The model under review builds one solid part; all positions refer to its coordinate system, in mm. A direction names the side the tool comes from. Round coordinates to 2 decimals unless told otherwise and drop trailing zeros. Loops run counter-clockwise (first coordinate to the right, second up) from the corner with the lowest first, then second, coordinate; pieces in that order, holes last. Notation, with made-up numbers: (54.25, -19.5) -> (63.25, -19.5) arc R19 ccw to (63.25, 9.5) -> close; hole circle Ø11 at (32.5, 19.25). An arc over 180 degrees is marked (long way). Write each question's results on one line, items separated by ' | '. Start each with the question number.
Item 1: Clearance check with a flat-ended pin moving along its axis: pin 1 Ø1.9 at (x, z) = (-10, 22) entering from -Y. State where the tip first meets the part, or that it passes through.
Item 2: Mouldability with a two-part tool opening along X and no side actions: class faces 1 (the flat face through (30, 1, 0)), 2 (the flat face through (0, 1, -12.05)), 3 (the cylindrical face through (-26.58, 1.42, -21.39)) as pulls with the +X half, pulls with the -X half, needs draft (parallel to the pull), parting line crosses it, or undercut.
Item 3: We need section B-B (x = 10). Give the boundary of the cut face in (y, z), and give its area (3 significant figures).
Item 4: We need section D-D (x = -1). Give the boundary of the cut face in (y, z), and give its area (3 significant figures).
Item 5: Tool access review of faces 4 (the cylindrical face through (15.009, 1.38, 11.537)), 5 (the flat face through (0, 1, 25)): name each direction out of +Z, -Z, +X, -X, +Y, -Y from which nothing blocks a thin tool from reaching the whole face with its end or side.
Item 6: For L1, parallel to Z at x = 10, y = 1; L2, parallel to Z at x = -7, y = 0.35; L3, parallel to X at y = 0.1, z = 21, list the stretches that pass through material, from the lowest coordinate up. Write a range as from..to.
Item 7: We need section A-A (z = 8). Give the boundary of the cut face in (x, y), and give its area (3 significant figures).
Item 8: We need section C-C (y = 0.45). Give the number of separate pieces and of enclosed holes in the cut face, and give its area (3 significant figures).
from build123d import *

# Parameters (mm, degrees)
SKETCH_1_W          = 60
SKETCH_1_H          = 50
SKETCH_1_W_2        = 29.5
SKETCH_1_H_2        = 22.5
EXTRUDE_1_DEPTH     = 2.8
SKETCH_8_R          = 1.55
CUT_EXTRUDE_2_DEPTH = 10
FILLET_1_R          = 1
FILLET_2_R          = 12
CUT_EXTRUDE_3_DEPTH = 10


with BuildPart() as part:
    # 草图1 → 凸台-拉伸1 (new body)
    with BuildSketch(Plane(origin=(0, 0, 0), x_dir=(1, 0, 0), z_dir=(0, 1, 0))):
        Rectangle(SKETCH_1_W, SKETCH_1_H)
        Rectangle(SKETCH_1_W_2, SKETCH_1_H_2, mode=Mode.SUBTRACT)
    extrude(amount=EXTRUDE_1_DEPTH)

    # 草图8 → 切除-拉伸2 (cut)
    with BuildSketch(Plane.XZ):
        with Locations((27, 8)):
            Circle(SKETCH_8_R)
        with Locations((10, 22)):
            Circle(SKETCH_8_R)
        with Locations((-10, 22)):
            Circle(SKETCH_8_R)
        with Locations((-27, 8)):
            Circle(SKETCH_8_R)
        with Locations((-27, -8)):
            Circle(SKETCH_8_R)
        with Locations((-10, -22)):
            Circle(SKETCH_8_R)
        with Locations((10, -22)):
            Circle(SKETCH_8_R)
        with Locations((27, -8)):
            Circle(SKETCH_8_R)
    extrude(amount=-CUT_EXTRUDE_2_DEPTH, mode=Mode.SUBTRACT)

    # 圆角1
    fillet_1_edges = [part.edges().sort_by_distance(p)[0] for p in [
        (14.75, 1.4, 11.25),
        (14.75, 1.4, -11.25),
        (-14.75, 1.4, -11.25),
        (-14.75, 1.4, 11.25),
    ]]
    fillet(fillet_1_edges, radius=FILLET_1_R)

    # 圆角2
    fillet_2_edges = [part.edges().sort_by_distance(p)[0] for p in [
        (30, 1.4, 25),
        (-30, 1.4, 25),
        (-30, 1.4, -25),
        (30, 1.4, -25),
    ]]
    fillet(fillet_2_edges, radius=FILLET_2_R)

    # 草图9 → 切除-拉伸3 (cut)
    with BuildSketch(Plane.XZ):
        with BuildLine():
            Line((-13.75, 12.05), (13.75, 12.05))
            ThreePointArc((13.75, 12.05), (15.022792206, 11.522792206), (15.55, 10.25))
            Line((15.55, 10.25), (15.55, -10.25))
            ThreePointArc((15.55, -10.25), (15.022792206, -11.522792206), (13.75, -12.05))
            Line((13.75, -12.05), (-13.75, -12.05))
            ThreePointArc((-13.75, -12.05), (-15.022792206, -11.522792206), (-15.55, -10.25))
            Line((-15.55, -10.25), (-15.55, 10.25))
            ThreePointArc((-15.55, 10.25), (-15.022792206, 11.522792206), (-13.75, 12.05))
        make_face()
    extrude(amount=-CUT_EXTRUDE_3_DEPTH, mode=Mode.SUBTRACT)


solid = part.part
Here are the results:
1) pin 1: passes through
2) face 1: pulls with the +X half | face 2: undercut | face 3: pulls with the -X half
3) outline: (0, -25) -> (2.8, -25) -> (2.8, -23.55) -> (0, -23.55) -> close; (0, -20.45) -> (2.8, -20.45) -> (2.8, -12.05) -> (0, -12.05) -> close; (0, 12.05) -> (2.8, 12.05) -> (2.8, 20.45) -> (0, 20.45) -> close; (0, 23.55) -> (2.8, 23.55) -> (2.8, 25) -> (0, 25) -> close | area: 55.2 mm2
4) outline: (0, -25) -> (2.8, -25) -> (2.8, -12.05) -> (0, -12.05) -> close; (0, 12.05) -> (2.8, 12.05) -> (2.8, 25) -> (0, 25) -> close | area: 72.5 mm2
5) face 4: +Y, -Y | face 5: +Z, +X, -X, +Y, -Y
6) L1: z = -25..-23.55, -20.45..-12.05, 12.05..20.45, 23.55..25 | L2: z = -25..-12.05, 12.05..25 | L3: x = -26.94..-11.18, -8.82..8.82, 11.18..26.94
7) outline: (-30, 0) -> (-28.55, 0) -> (-28.55, 2.8) -> (-30, 2.8) -> close; (-25.45, 0) -> (-15.55, 0) -> (-15.55, 2.8) -> (-25.45, 2.8) -> close; (15.55, 0) -> (25.45, 0) -> (25.45, 2.8) -> (15.55, 2.8) -> close; (28.55, 0) -> (30, 0) -> (30, 2.8) -> (28.55, 2.8) -> close | area: 63.6 mm2
8) separate pieces: 1 | enclosed holes: 9 | area: 2,070 mm2
